Read the model definition and answer for the solid it produces. Units are mm, in the model's axes. Face numbers are marked on the shaded views. A direction names the side the tool comes from. Coordinates: 2 decimals unless noted, no trailing zeros. Order: outer loops, then holes, each group sorted by start corner. A loop starts at its lowest first (then second) coordinate and runs counter-clockwise, first axis right, second up. Notation, with made-up numbers: (-32, 24.25) - (26, 24.25) arc R28 ccw to (26, 44.25) - close; hole circle Ø3 at (-9, -14.5). An arc over 180 degrees is marked (long way). Write item = value, one per line.
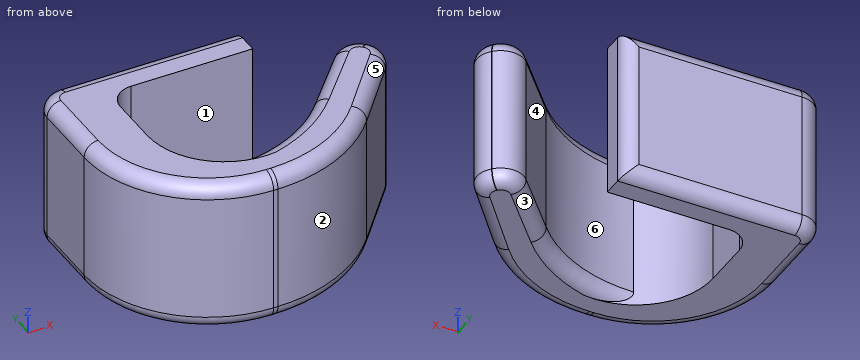
from build123d import *

# Parameters (mm, degrees)
SALIENTE_EXTRUIR1_DEPTH = 10
REDONDEO8_R             = 0.9


with BuildPart() as part:
    # Croquis2 → Saliente-Extruir1 (new body)
    with BuildSketch(Plane.XY):
        with BuildLine():
            Line((-5.744063225, 0), (5.744063225, 0))
            Line((5.744063225, 0), (5.744063225, -2.147495728))
            Line((5.744063225, -2.147495728), (-2.139285526, -2.147495728))
            ThreePointArc((-2.139285526, -2.147495728), (-3.199945698, -2.586835556), (-3.639285526, -3.647495728))
            Line((-3.639285526, -3.647495728), (-3.639285526, -6.880160463))
            ThreePointArc((-3.639285526, -6.880160463), (-2.897621881, -9.500574837), (-0.892656931, -11.34360278))
            ThreePointArc((-0.892656931, -11.34360278), (3.193809946, -10.470529341), (6.566719686, -8.003760473))
            Line((6.566719686, -8.003760473), (9.81244552, -4.368547538))
            ThreePointArc((9.81244552, -4.368547538), (10.916709754, -3.867642659), (12.03054225, -4.346894543))
            Line((12.03054225, -4.346894543), (12.051695209, -4.369674653))
            ThreePointArc((12.051695209, -4.369674653), (12.451992737, -5.351153846), (12.103519704, -6.352206325))
            Line((12.103519704, -6.352206325), (8.710612857, -10.412366821))
            ThreePointArc((8.710612857, -10.412366821), (5.272528505, -13.058798712), (1.037181306, -14))
            Line((1.037181306, -14), (0.755936775, -14))
            ThreePointArc((0.755936775, -14), (-4.900917475, -11.656854249), (-7.244063225, -6))
            Line((-7.244063225, -6), (-7.244063225, -1.5))
            ThreePointArc((-7.244063225, -1.5), (-6.804723397, -0.439339828), (-5.744063225, 0))
        make_face()
    extrude(amount=SALIENTE_EXTRUIR1_DEPTH)

    # Redondeo8
    redondeo8_edges = [part.edges().sort_by_distance(p)[0] for p in [
        (-6.804723397, -0.439339828, 10),
        (-7.244063225, -3.75, 10),
        (3.193809946, -10.470529341, 0),
        (8.189582603, -6.186154005, 0),
        (10.916709754, -3.867642659, 0),
        (12.041118729, -4.358284598, 0),
        (12.451992737, -5.351153846, 0),
        (10.40706628, -8.382286573, 0),
        (5.272528505, -13.058798712, 0),
        (-4.900917475, -11.656854249, 10),
        (0.89655904, -14, 0),
        (-4.900917475, -11.656854249, 0),
        (-7.244063225, -3.75, 0),
        (-6.804723397, -0.439339828, 0),
        (0, 0, 0),
        (0.89655904, -14, 10),
        (5.272528505, -13.058798712, 10),
        (5.744063225, 0, 5),
        (10.40706628, -8.382286573, 10),
        (12.451992737, -5.351153846, 10),
        (12.041118729, -4.358284598, 10),
        (10.916709754, -3.867642659, 10),
        (8.189582603, -6.186154005, 10),
        (3.193809946, -10.470529341, 10),
        (0, 0, 10),
    ]]
    fillet(redondeo8_edges, radius=REDONDEO8_R)


solid = part.part
1) For the marked faces 1, 2 and 3, determine the directions among +Z, -Z, +X, -X, +Y, -Y from which every point of the face is accessible in a straight line to the end or side of a thin tool.
Returned:
face_1 = +Z, -Z, +X
face_2 = +Z, -Z, +X, -Y
face_3 = -Z, +Y
2) Flat-ended cylindrical pins translate along their axes: pin 1 Ø1.4 at (y, z) = (-1.5, 7) entering from +X; pin 2 Ø1 at (x, z) = (6, 2.5) entering from -Y; pin 3 Ø3 at (x, z) = (-2.5, 6.5) entering from -Y. Find the tip coordinate at first contact, or state that the pin passes through.
Returned:
pin_1 = 5.74
pin_2 = -12.95
pin_3 = -13.8
3) The part is cut by section B-B (y = -3). Determine the outline of the cut face in (x, z).
Returned:
outline = (-7.24, 0.9) arc R0.9 ccw to (-6.34, 0) - (-3.49, 0) - (-3.49, 10) - (-6.34, 10) arc R0.9 ccw to (-7.24, 9.1) - close
4) Determine the mould class of the marked faces 4, 5 and 6 for opening direction Y: pulls with the +Y half, pulls with the -Y half, needs draft (parallel to the pull), parting line crosses it, or undercut.
Returned:
face_4 = pulls with the +Y half
face_5 = pulls with the -Y half
face_6 = undercut
5) Straight lines are drawn through the part: line 1 along X through (y, z) = (-6, 1.5); line 2 along Y through (x, z) = (5, 9.25); line 3 along X through (y, z) = (-4.75, 9.75). For each, find the intervals that lie inside material, in ascending order. Write a range as from..to.
Returned:
line_1 = -7.24..-3.64, 8.36..12.32
line_2 = -13.17..-9.44, -2.15..-0.01
line_3 = -6.97..-3.64, 9.84..11.99
